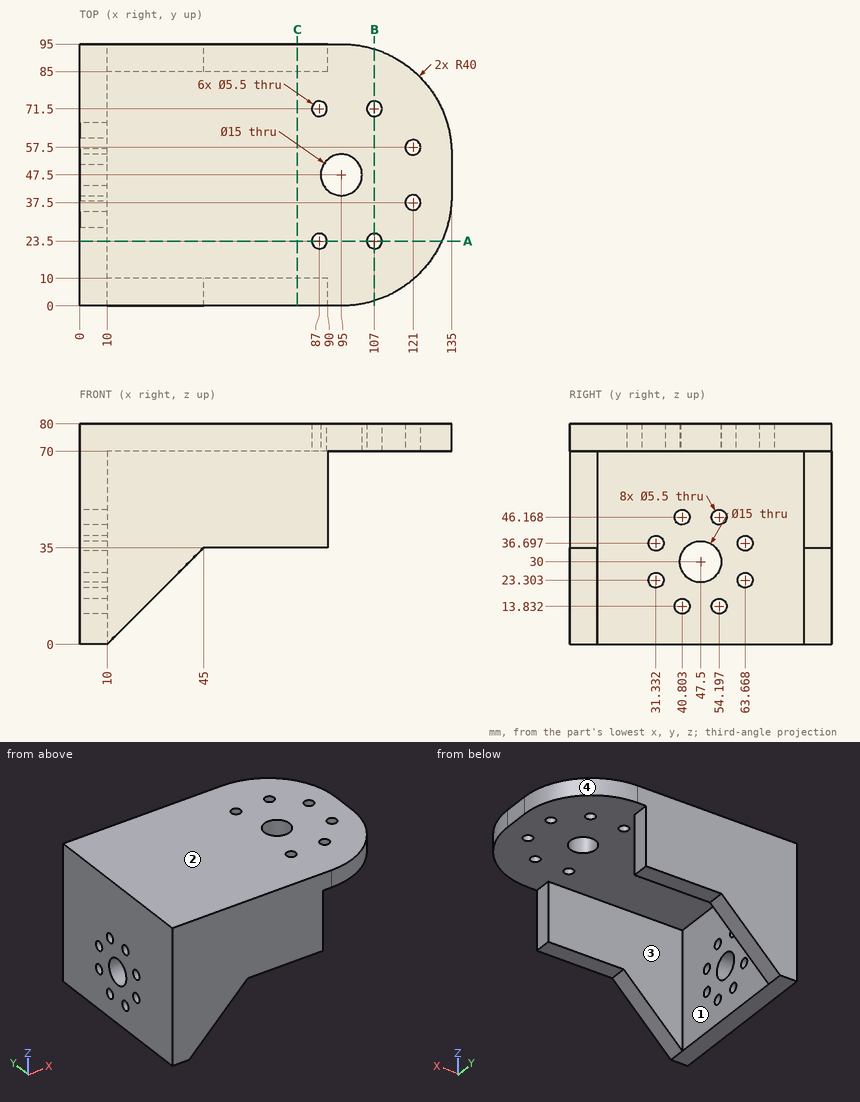
Check sheet for the drawn part. Datum: minimum x, y, z corner. Units: mm. Round coordinates to 2 decimals unless told otherwise and drop trailing zeros. Order: outer loops, then holes, each group sorted by start corner. A loop starts at its lowest first (then second) coordinate and runs counter-clockwise, first axis right, second up. Notation, with made-up numbers: M -26,-37.75 L -2,-37.75 A28 ccw -2,-5.75 Z; hole C -20.75,3 d4. An arc over 180 degrees is marked long. Write each question's results on one line, items separated by ' | '. Start each with the question number.
1. Draft check along Y on the marked faces 1, 2, 3 and 4. Enter one of: pulls with the +Y half, pulls with the -Y half, needs draft (parallel to the pull), parting line crosses it, or undercut.
2. Cross-section at A-A on y = 23.5. Record the boundary of the cut face in (x, z).
3. Cross-section at C-C on x = 79. Record the boundary of the cut face in (y, z), plus the area to 3 significant figures.
4. Cross-section at B-B on x = 107. Record the boundary of the cut face in (y, z), plus the area to 3 significant figures.
5. Go/stop test with flat-tipped pins: P1, Ø5, axis at x = 107, y = 71.5, coming from the +Z side; P2, Ø3, axis at y = 92.5, z = 48.5, coming from the +X side; P3, Ø6.5, axis at y = 40.8, z = 46.17, coming from the -X side; P4, Ø6.5, axis at x = 87, y = 23.5, coming from the -Z side. Record where each tip stops, or that it passes through.
6. Material ranges on L1, parallel to Y at x = 73, z = 66; L2, parallel to Z at x = 73.5, y = 18.5; L3, parallel to X at y = 34, z = 45.5, recorded low to high. Write a range as from..to.
Resolved:
1) face 1: undercut | face 2: needs draft | face 3: undercut | face 4: pulls with the +Y half
2) outline: M 0,0 L 10,0 L 10,70 L 84.25,70 L 84.25,80 L 0,80 Z; M 89.75,70 L 104.25,70 L 104.25,80 L 89.75,80 Z; M 109.75,70 L 131.44,70 L 131.44,80 L 109.75,80 Z
3) outline: M 0,35 L 10,35 L 10,70 L 85,70 L 85,35 L 95,35 L 95,80 L 0,80 Z | area: 1,650 mm2
4) outline: M 1.84,70 L 20.75,70 L 20.75,80 L 1.84,80 Z; M 26.25,70 L 68.75,70 L 68.75,80 L 26.25,80 Z; M 74.25,70 L 93.16,70 L 93.16,80 L 74.25,80 Z | area: 803 mm2
5) P1: through | P2: x = 90 | P3: x = 0 | P4: z = 70
6) L1: 0..10, 85..95 | L2: 70..80 | L3: 0..10
